```python
from build123d import *

# Parameters (mm, degrees)
EXTRUDE_1_DEPTH     = 8
CUT_EXTRUDE_START   = -5
SKETCH_2_R          = 3
CUT_EXTRUDE_1_DEPTH = 10
SKETCH_2_3_R        = 1.7
CUT_EXTRUDE_2_DEPTH = 5
SKETCH_3_R          = 1.7
CUT_EXTRUDE_4_DEPTH = 5
SKETCH_3_3_R        = 3
CUT_EXTRUDE_3_DEPTH = 10
CHAMFER_1_SIZE      = 0.5


with BuildPart() as part:
    # 草图1 → 凸台-拉伸1 (new body)
    with BuildSketch(Plane.XY):
        with BuildLine():
            Line((-7.824326088, 23.005235362), (-7.824326088, 15.505235362))
            ThreePointArc((-7.824326088, 15.505235362), (-0.324326088, 8.005235362), (-7.824326088, 0.505235362))
            Line((-7.824326088, 0.505235362), (-7.824326088, -6.994764638))
            ThreePointArc((-7.824326088, -6.994764638), (7.175673912, 8.005235362), (-7.824326088, 23.005235362))
        make_face()
    extrude(amount=EXTRUDE_1_DEPTH)

    # 草图2 → 切除-拉伸1 (cut)
    with BuildSketch(Plane.ZY.offset(7.824326088).offset(CUT_EXTRUDE_START)):
        with Locations((4, 19.255235362)):
            Circle(SKETCH_2_R)
    extrude(amount=-CUT_EXTRUDE_1_DEPTH, mode=Mode.SUBTRACT)

    # 草图2<3> → 切除-拉伸2 (cut)
    with BuildSketch(Plane.ZY.offset(7.824326088)):
        with Locations((4, 19.255235362)):
            Circle(SKETCH_2_3_R)
    extrude(amount=-CUT_EXTRUDE_2_DEPTH, mode=Mode.SUBTRACT)

    # 草图3 → 切除-拉伸4 (cut)
    with BuildSketch(Plane.ZY.offset(7.824326088)):
        with Locations((4, -3.244764638)):
            Circle(SKETCH_3_R)
    extrude(amount=-CUT_EXTRUDE_4_DEPTH, mode=Mode.SUBTRACT)

    # 草图3<3> → 切除-拉伸3 (cut)
    with BuildSketch(Plane.ZY.offset(7.824326088).offset(CUT_EXTRUDE_START)):
        with Locations((4, -3.244764638)):
            Circle(SKETCH_3_3_R)
    extrude(amount=-CUT_EXTRUDE_3_DEPTH, mode=Mode.SUBTRACT)

    # 倒角1
    chamfer_1_edges = [part.edges().sort_by_distance(p)[0] for p in [
        (7.175673912, 8.005235362, 8),
        (-0.324326088, 8.005235362, 8),
        (7.175673912, 8.005235362, 0),
        (-0.324326088, 8.005235362, 0),
    ]]
    chamfer(chamfer_1_edges, length=CHAMFER_1_SIZE)


solid = part.part
```
Could you check a few things on this model? Use its own coordinates, in mm. A direction names the side the tool comes from. Round coordinates to 2 decimals unless told otherwise and drop trailing zeros. Loops run counter-clockwise (first coordinate to the right, second up) from the corner with the lowest first, then second, coordinate; pieces in that order, holes last. Notation, with made-up numbers: (-24, 58.5) - (0, 58.5) arc R22 ccw to (0, 93.5) - close; hole circle Ø9 at (-22, 5.25). An arc over 180 degrees is marked (long way). Answer as CSV lines item,"result".
1. On a 3-axis mill with a long thin cutter (end or side, diameter ignored), from which of +Z, -Z, +X, -X, +Y, -Y can I reach the whole of each face in a straight line? I mean faces 1 (the face through (-5.359, 17.747, 4.784)), 2 (the face through (-2.824, 17.9, 5.3)). Say none if no direction works.
Filled in:
face 1,"+X, -X"
face 2,"+X"
2. I want a section at A-A on z = 4. List the corners of the cut face in (x, y) for me.
Filled in:
outline,"(-7.82, -6.99) arc R15 ccw to (-2.82, -6.14) - (-2.82, -4.94) - (-7.82, -4.94) - close; (-7.82, -1.54) - (-2.82, -1.54) - (-2.82, -0.24) - (4.7, -0.24) arc R15 ccw to (4.7, 16.26) - (-2.82, 16.26) - (-2.82, 17.56) - (-7.82, 17.56) - (-7.82, 15.51) arc R7.5 cw to (-7.82, 0.51) - close; (-7.82, 20.96) - (-2.82, 20.96) - (-2.82, 22.15) arc R15 ccw to (-7.82, 23.01) - close"
3. Please list where these lines run through material, in increasing order: line 1 along Y through (x, z) = (-3.8, 4); line 2 along Y through (x, z) = (-4, 5); line 3 along Y through (x, z) = (-1.5, 2.25). Write a range as [from, to].
Filled in:
line 1,"y = [-6.44, -4.94], [-1.54, 1.68], [14.33, 17.56], [20.96, 22.46]"
line 2,"y = [-6.5, -4.62], [-1.87, 1.55], [14.46, 17.88], [20.63, 22.51]"
line 3,"y = [-0.81, 3.97], [12.04, 16.82]"
4. For pin 1 Ø1.5 at (x, z) = (-4, 6) entering from +Y; pin 2 Ø2 at (x, z) = (-1.5, 6) entering from -Y; pin 3 Ø1 at (x, y) = (-4.5, 1.5) entering from -Z; pin 4 Ø3 at (y, z) = (-3.24, 4) entering from -X, each with a flat end and sliding along its axis, tell me the tip position at first contact or that it passes through.
Filled in:
pin 1,"stops at y = 22.69"
pin 2,"stops at y = -6.02"
pin 3,"stops at z = 0.19"
pin 4,"passes through"
5. I want a section at B-B on z = 1.5. List the corners of the cut face in (x, y) for me, then the cut area to 3 significant figures.
Filled in:
outline,"(-7.82, -6.99) arc R15 ccw to (-0.18, -4.9) - (-2.82, -4.9) - (-2.82, -1.59) - (3.71, -1.59) arc R15 ccw to (3.71, 17.6) - (-2.82, 17.6) - (-2.82, 20.91) - (-0.18, 20.91) arc R15 ccw to (-7.82, 23.01) - (-7.82, 15.51) arc R7.5 cw to (-7.82, 0.51) - close"
area,"233 mm^2"
6. We'd pull the mould along Z, two halves only. Please class faces 3 (the face through (-2.824, -4.5, 2.6)), 4 (the face through (6.81, 7.68, 7.86)), 5 (the face through (-0.184, 8.173, 0.358)): +Z half, -Z half, draft (parallel to the pull), parting line (faces both ways), or undercut.
Filled in:
face 3,"undercut"
face 4,"+Z half"
face 5,"-Z half"
